Work out the finished part from the listing and answer in its coordinate system (mm). A direction names the side the tool comes from. Give positions to 0.01 mm unless a question says otherwise; leave off trailing zeros. Order: outer loops, then holes, each group sorted by start corner. A loop starts at its lowest first (then second) coordinate and runs counter-clockwise, first axis right, second up. Notation, with made-up numbers: (11, 6) - (30, 6) arc R10 ccw to (30, 20) - close; hole circle Ø10 at (-1, -17). An arc over 180 degrees is marked (long way). Put each result on its own line as item: value.
```python
from build123d import *

# Parameters (mm, degrees)
BOSS_EXTRUDE1_DEPTH   = 100
M5X0_8_TAPPED_HOLE1_D = 4.2


with BuildPart() as part:
    # Sketch1 → Boss-Extrude1 (new body)
    with BuildSketch(Plane.XY):
        Polygon((2.25, 0), (-2.25, 0), (-4.65, 2.4), (-4.65, 3.4), (-2.9, 3.4), (-2.9, 4.4), (2.9, 4.4), (2.9, 3.4), (4.65, 3.4), (4.65, 2.4), align=None)
    extrude(amount=BOSS_EXTRUDE1_DEPTH)

    # M5x0.8 Tapped Hole1 (through all)
    with Locations(Plane(origin=(0, 4.4, 0), x_dir=(1, 0, 0), z_dir=(0, 1, 0))):
        with Locations((0, -10), (0, -40), (0, -60), (0, -90)):
            Hole(M5X0_8_TAPPED_HOLE1_D / 2)


solid = part.part
```
(1) Section B-B, the plane z = 10 is taken. Write down the section's boundary in (x, y).
Geometry check:
outline: (-4.65, 2.4) - (-2.25, 0) - (-2.1, 0) - (-2.1, 4.4) - (-2.9, 4.4) - (-2.9, 3.4) - (-4.65, 3.4) - close; (2.1, 0) - (2.25, 0) - (4.65, 2.4) - (4.65, 3.4) - (2.9, 3.4) - (2.9, 4.4) - (2.1, 4.4) - close
(2) Section A-A, the plane x = 0 is taken. Write down the section's boundary in (y, z).
Geometry check:
outline: (0, 0) - (4.4, 0) - (4.4, 7.9) - (0, 7.9) - close; (0, 12.1) - (4.4, 12.1) - (4.4, 37.9) - (0, 37.9) - close; (0, 42.1) - (4.4, 42.1) - (4.4, 57.9) - (0, 57.9) - close; (0, 62.1) - (4.4, 62.1) - (4.4, 87.9) - (0, 87.9) - close; (0, 92.1) - (4.4, 92.1) - (4.4, 100) - (0, 100) - close
(3) Section C-C, the plane y = 0.95 is taken. Write down the section's boundary in (x, z).
Geometry check:
outline: (-3.2, 0) - (3.2, 0) - (3.2, 100) - (-3.2, 100) - close; hole circle Ø4.2 at (0, 10); hole circle Ø4.2 at (0, 40); hole circle Ø4.2 at (0, 60); hole circle Ø4.2 at (0, 90)
(4) Given pin 1 (4 mm diameter, centred on x = 0, z = 60, fed in from +Y); pin 2 (1.1 mm diameter, centred on y = 4, z = 44, fed in from +X); pin 3 (1.9 mm diameter, centred on x = 3.5, z = 31.5, fed in from +Y); pin 4 (0.5 mm diameter, centred on x = -4, z = 25.5, fed in from +Y), each flat-ended and moving along its own axis, determine where each tip first touches the part or whether it passes through.
Geometry check:
pin 1: passes through
pin 2: stops at x = 2.9
pin 3: stops at y = 4.4
pin 4: stops at y = 3.4
(5) Straight lines are drawn through the part: line 1 (Z direction, x = 0, y = 1.8); line 2 (X direction, y = 2, z = 60); line 3 (X direction, y = 3.9, z = 69.5). For each, find the intervals that lie inside material, in ascending order.
Geometry check:
line 1: z = 0 to 7.9, 12.1 to 37.9, 42.1 to 57.9, 62.1 to 87.9, 92.1 to 100
line 2: x = -4.25 to -2.1, 2.1 to 4.25
line 3: x = -2.9 to 2.9
(6) A tool of negligible diameter and unlimited length cuts with its end or side. For faces 1 (the face through (-4, 3.4, 49)), 2 (the face through (0, 0, 49)), 3 (the face through (4, 3.4, 49)), from which of +Z, -Z, +X, -X, +Y, -Y can it reach the whole face along a straight path? Write none if from no direction.
Geometry check:
face 1: +Z, -Z, -X, +Y
face 2: +Z, -Z, +X, -X, -Y
face 3: +Z, -Z, +X, +Y
(7) Determine the mould class of faces 4 (the face through (-3.43, 1.18, 49.3)), 5 (the face through (0, 2, 0)), 6 (the face through (3.47, 1.22, 49.3)), 7 (the face through (0.46, 2.17, 62.05)) for opening direction X: pulls with the +X half, pulls with the -X half, needs draft (parallel to the pull), parting line crosses it, or undercut.
Geometry check:
face 4: pulls with the -X half
face 5: needs draft
face 6: pulls with the +X half
face 7: undercut
(8) Section D-D, the plane z = 85.5 is taken. Write down the section's boundary in (x, y), then the cut area to 3 significant figures.
Geometry check:
outline: (-4.65, 2.4) - (-2.25, 0) - (2.25, 0) - (4.65, 2.4) - (4.65, 3.4) - (2.9, 3.4) - (2.9, 4.4) - (-2.9, 4.4) - (-2.9, 3.4) - (-4.65, 3.4) - close
area: 31.7 mm²
